from build123d import *

# Parameters (mm, degrees)
SKETCH1_W           = 7.83
SKETCH1_H           = 7.83
BOSS_EXTRUDE1_DEPTH = 3.17
SKETCH2_R           = 2.325
BOSS_EXTRUDE2_DEPTH = 1.86
SHELL2_T            = -1.45


with BuildPart() as part:
    # Sketch1 → Boss-Extrude1 (new body)
    with BuildSketch(Plane(origin=(0, 0, 0), x_dir=(1, 0, 0), z_dir=(0, 1, 0))):
        Rectangle(SKETCH1_W, SKETCH1_H)
    extrude(amount=-BOSS_EXTRUDE1_DEPTH)

    # Sketch2 → Boss-Extrude2 (add)
    with BuildSketch(Plane(origin=(0, 0, 0), x_dir=(1, 0, 0), z_dir=(0, 1, 0))):
        with Locations(Location((0, 0, 0), (0, 0, 270))):
            Circle(SKETCH2_R)
    extrude(amount=BOSS_EXTRUDE2_DEPTH)

    # Shell2
    shell2_openings = [part.faces().sort_by_distance(p)[0] for p in [
        (0, -3.17, 0),
    ]]
    offset(amount=SHELL2_T, openings=shell2_openings, kind=Kind.INTERSECTION)


solid = part.part
Verification items for the finished model (mm, model axes). A direction names the side the tool comes from. Give positions to 0.01 mm unless a question says otherwise; leave off trailing zeros. Order: outer loops, then holes, each group sorted by start corner. A loop starts at its lowest first (then second) coordinate and runs counter-clockwise, first axis right, second up. Notation, with made-up numbers: M 78,20.5 L 135,20.5 A15 cw 135,43.5 Z; hole C 56,71.25 d2. An arc over 180 degrees is marked long. Use one line per item in the form item = value. Start each with the question number.
Q1. Section check A-A (y = -2.45). Enter the section's corners in (x, z) (3 decimals).
Q2. Section check B-B (x = 0). Enter the section's corners in (y, z) (3 decimals), then the cut area to 3 significant figures.
Q3. Mould release check, pull along Z, two halves, no side actions. Record for faces 4 (the flat face through (3.915, -2, 0)), 5 (the flat face through (0, 0.41, 0)), 6 (the flat face through (0, -2, -3.915)): +Z half, -Z half, draft (parallel to the pull), parting line (faces both ways), or undercut.
Q4. Go/stop test with flat-tipped pins: pin 1 Ø4 at (x, z) = (-0.5, 0.5) entering from -Y; pin 2 Ø1.4 at (x, z) = (0, 0) entering from -Y; pin 3 Ø1.5 at (y, z) = (1, -1.5) entering from -X. Record where each tip stops, or that it passes through.
Q5. Access from +Z, -Z, +X, -X, +Y, -Y to the whole of each face (thin tool, end or side, straight path). Record for faces 1 (the flat face through (-3.915, -2, 0)), 2 (the flat face through (2.465, -2, 0)), 3 (the cylindrical face through (0.698, 0.917, 2.218)).
Q6. Scan lines: line 1 along Z through (x, y) = (0, -0.5) (3 decimals); line 2 along Y through (x, z) = (-1.75, 3). Record each from-to range of solid material in increasing order. Write a range as [from, to].
Q7. Section check D-D (y = 0.8). Enter the section's corners in (x, z) (3 decimals).
Q8. Section check C-C (z = 0). Enter the section's corners in (x, y) (3 decimals), then the cut area to 3 significant figures.
Evaluation:
q1.outline = M -3.915,-3.915 L 3.915,-3.915 L 3.915,3.915 L -3.915,3.915 Z; hole M -2.465,-2.465 L 2.465,-2.465 L 2.465,2.465 L -2.465,2.465 Z
q2.outline = M -3.17,-3.915 L 0,-3.915 L 0,-2.325 L 1.86,-2.325 L 1.86,2.325 L 0,2.325 L 0,3.915 L -3.17,3.915 L -3.17,2.465 L -1.45,2.465 L -1.45,0.875 L 0.41,0.875 L 0.41,-0.875 L -1.45,-0.875 L -1.45,-2.465 L -3.17,-2.465 Z
q2.area = 21.7 mm2
q3.face_4 = draft
q3.face_5 = undercut
q3.face_6 = -Z half
q4.pin_1 = -3.17
q4.pin_2 = 0.41
q4.pin_3 = -2.2
q5.face_1 = +Z, -Z, -X, +Y, -Y
q5.face_2 = -Y
q5.face_3 = +Y
q6.line_1 = [-3.915, -0.875], [0.875, 3.915]
q6.line_2 = [-3.17, 0]
q7.outline = C 0,0 d4.65
q8.outline = M -3.915,-3.17 L -2.465,-3.17 L -2.465,-1.45 L -0.875,-1.45 L -0.875,0.41 L 0.875,0.41 L 0.875,-1.45 L 2.465,-1.45 L 2.465,-3.17 L 3.915,-3.17 L 3.915,0 L 2.325,0 L 2.325,1.86 L -2.325,1.86 L -2.325,0 L -3.915,0 Z
q8.area = 21.7 mm2
